Autodesk Inventor part; units mm, degrees
ref_plane "YZ Plane" through (0, 0, 0) normal (1, 0, 0) x (0, 1, 0)
ref_plane "XZ Plane" through (0, 0, 0) normal (0, 1, 0) x (-1, 0, 0)
ref_plane "XY Plane" through (0, 0, 0) normal (0, 0, 1) x (1, 0, 0)
sketch "Sketch1" plane through (0, 0, 0) normal (0, 0, 1) x (1, 0, 0)
  line L0 (0, 0) -> (124, 0)
  line L1 (124, 0) -> (124, 124)
  line L2 (124, 124) -> (0, 124)
  line L3 (0, 124) -> (0, 0)
  dimension "d0" = 124
  dimension "d1" = 124
extrude "Extrusion1" add sketch "Sketch1" along normal blind 10
sketch "Sketch2" plane through (0, 0, 10) normal (0, 0, 1) x (1, 0, 0)
  line L0 (124, 0) -> (124, 124)
  line L1 (124, 124) -> (79.5, 124)
  line L2 (79.5, 124) -> (79.5, 6)
  line L3 (79.5, 6) -> (124, 6)
  line L4 (124, 6) -> (124, 124)
  point P0 (0, 0)
  dimension "d4" = 44.5
  dimension "d5" = 118
extrude "Extrusion2" cut sketch "Sketch2" against normal through all
sketch "Sketch3" plane through (0, 0, 10) normal (0, 0, 1) x (1, 0, 0)
  line L0 (0, 124) -> (0, 0)
  line L1 (0, 82) -> (-10, 82)
  line L2 (-10, 82) -> (-10, 42)
  line L3 (-10, 42) -> (0, 42)
  line L4 (0, 42) -> (0, 82)
  circle A0 centre (-5, 62) radius 2.5
  line L5 (0, 0) -> (124, 0)
  line L6 (42, 0) -> (82, 0)
  line L7 (82, 0) -> (82, -10)
  line L8 (82, -10) -> (42, -10)
  line L9 (42, -10) -> (42, 0)
  circle A1 centre (62, -5) radius 2.5
  point P0 (-10, 62)
  point P1 (0, 62)
  point P2 (-5, 82)
  point P3 (62, -10)
  point P4 (62, 0)
  point P5 (62, 0)
  point P6 (42, -5)
  dimension "d8" = 10
  dimension "d9" = 40
  dimension "d10" = 5
  dimension "d11" = 40
  dimension "d12" = 10
  dimension "d13" = 5
extrude "Extrusion3" add sketch "Sketch3" against normal blind 5
sketch "Sketch5" plane through (0, 0, 10) normal (0, 0, 1) x (1, 0, 0)
  line L0 (0, 124) -> (0, 82)
  line L1 (0, 124) -> (79.5, 124)
  line L2 (79.5, 124) -> (79.5, 119)
  line L3 (79.5, 119) -> (0, 119)
  line L4 (0, 119) -> (0, 124)
  line L5 (79.5, 6) -> (79.5, 124)
  point P0 (0, 0)
  dimension "d19" = 5
extrude "Extrusion5" cut sketch "Sketch5" against normal through all
properties part number "TC004" material "ABS Plastic"
Could you check a few things on this model? Use its own coordinates, in mm. A direction names the side the tool comes from. Coordinates: 2 decimals unless noted, no trailing zeros. Loops run counter-clockwise (first coordinate to the right, second up) from the corner with the lowest first, then second, coordinate; pieces in that order, holes last.
1) Imagine slicing it at C-C (z = 7.25). List the corners of the cut face in (x, y) for me, and give its area (3 significant figures).
Reported:
outline: (-10, 42) - (0, 42) - (0, 0) - (42, 0) - (42, -10) - (82, -10) - (82, 0) - (124, 0) - (124, 6) - (79.5, 6) - (79.5, 119) - (0, 119) - (0, 82) - (-10, 82) - close; hole circle Ø5 at (-5, 62); hole circle Ø5 at (62, -5)
area: 10,500 mm2
2) Will these pins go through, and if not, where does the flat tip stop? pin 1 Ø5 at (x, y) = (-7, 63) entering from -Z; pin 2 Ø3 at (x, y) = (62, -5) entering from +Z; pin 3 Ø4 at (x, z) = (-5.5, 7.5) entering from +Y; pin 4 Ø2.5 at (y, z) = (-7, 7) entering from -X.
Reported:
pin 1: stops at z = 5
pin 2: passes through
pin 3: stops at y = 82
pin 4: stops at x = 42
3) Please list where these lines run through material, in increasing order: line 1 along Y through (x, z) = (-5, 8.3); line 2 along Y through (x, z) = (62, 7); line 3 along X through (y, z) = (71.5, 3).
Reported:
line 1: y = 42 to 59.5, 64.5 to 82
line 2: y = -10 to -7.5, -2.5 to 119
line 3: x = 0 to 79.5
4) Imagine slicing it at B-B (y = 62). List the corners of the cut face in (x, z) for me, and give its area (3 significant figures).
Reported:
outline: (-10, 5) - (-7.5, 5) - (-7.5, 10) - (-10, 10) - close; (-2.5, 5) - (0, 5) - (0, 0) - (79.5, 0) - (79.5, 10) - (-2.5, 10) - close
area: 820 mm2
5) Which directions (+Z, -Z, +X, -X, +Y, -Y) give clear straight access to the entire face, cutting with the end or side of a thin tool? Please do faces 1 (the face through (42, -5, 8)), 2 (the face through (101, 6, 5)), 3 (the face through (62, -2, 5)), 4 (the face through (-8, 62, 5)).
Reported:
face 1: +Z, -Z, -X, -Y
face 2: +Z, -Z, +X, +Y
face 3: -Z, +X, -X, -Y
face 4: -Z, -X, +Y, -Y
6) Thinking about a two-plate mould opening in X: for faces 5 (the face through (64.385, -4.249, 7.535)), 6 (the face through (-2.615, 62.751, 7.535)), 7 (the face through (82, -5, 8)), 8 (the face through (61, 0, 4)), which applies, released by +X, released by -X, zero draft, split by the parting line, or undercut?
Reported:
face 5: undercut
face 6: undercut
face 7: released by +X
face 8: zero draft
7) Imagine slicing it at A-A (x = -5). List the corners of the cut face in (y, z) for me.
Reported:
outline: (42, 5) - (59.5, 5) - (59.5, 10) - (42, 10) - close; (64.5, 5) - (82, 5) - (82, 10) - (64.5, 10) - close
